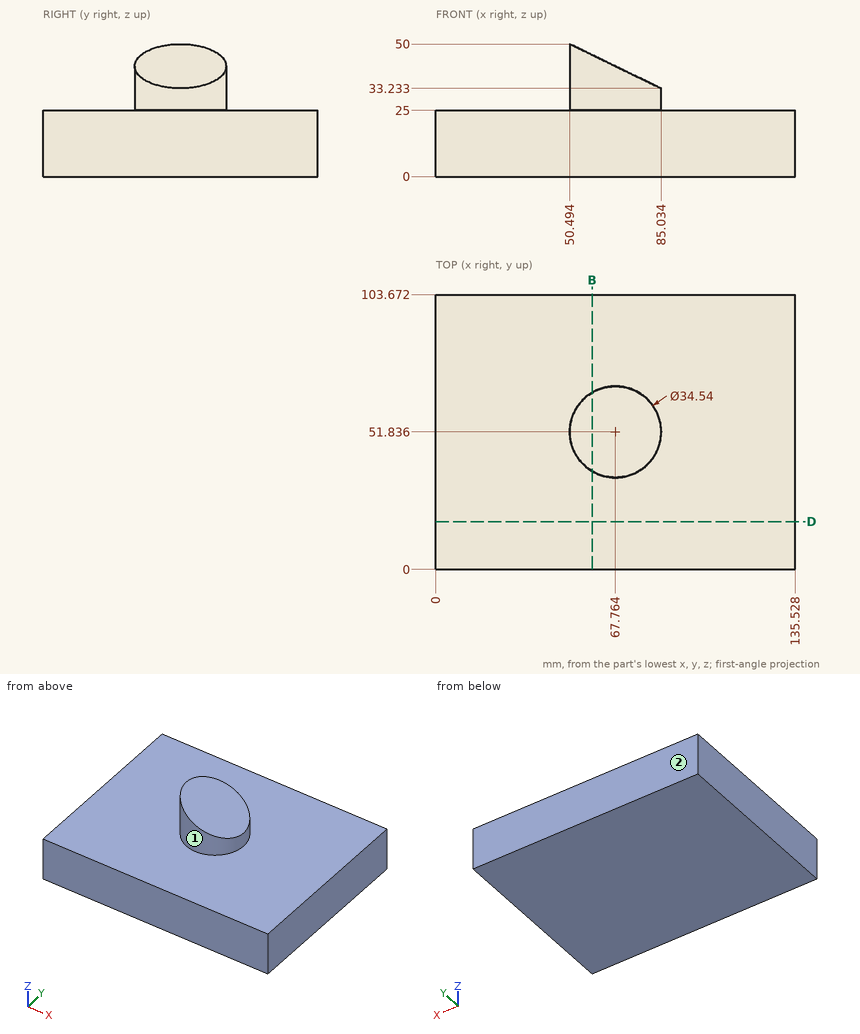
Job drawing, mm, ordinate dimensions from the low corner. One solid piece. A direction names the side the tool comes from. Round coordinates to 2 decimals unless told otherwise and drop trailing zeros. Order: outer loops, then holes, each group sorted by start corner. A loop starts at its lowest first (then second) coordinate and runs counter-clockwise, first axis right, second up. Notation, with made-up numbers: (69, 65.5) -> (104, 65.5) arc R26 cw to (104, 103.5) -> close; hole circle Ø8 at (65, 28). An arc over 180 degrees is marked (long way). Write item = value, one per line.
(1) 3-axis set-ups, long thin cutter, end or side, ignore diameter. For the marked faces 1 and 2: which of +Z, -Z, +X, -X, +Y, -Y reach the whole face in a straight line?
Answers follow:
face_1 = +Z
face_2 = +Z, -Z, +X, -X, +Y
(2) Cut at D-D (y = 18). Write the cut outline in (x, z), plus the area to 3 significant figures.
Answers follow:
outline = (0, 0) -> (135.53, 0) -> (135.53, 25) -> (0, 25) -> close
area = 3,390 mm²
(3) Flat gauge pins, fed straight in: P1, Ø2, axis at x = 94.5, z = 26.5, coming from the +Y side; P2, Ø1, axis at x = 107, y = 25, coming from the +Z side. Where does each tip first touch, or does it go through?
Answers follow:
P1 = through
P2 = 25
(4) Drill centre lines: L1, parallel to Z at x = 21, y = 19; L2, parallel to Y at x = 67.5, z = 37; L3, parallel to X at y = 57.5, z = 27. Where is each one in solid material? Low to high.
Answers follow:
L1 = 0 to 25
L2 = 34.57 to 69.1
L3 = 51.45 to 84.08
(5) Cut at B-B (x = 59). Write the cut outline in (y, z) (1 decimal), plus the area to 3 significant figures.
Answers follow:
outline = (0, 0) -> (103.7, 0) -> (103.7, 25) -> (66.7, 25) -> (66.7, 45.9) -> (37, 45.9) -> (37, 25) -> (0, 25) -> close
area = 3,210 mm²
